from build123d import *

# Parameters (mm, degrees)
F8_DEPTH  = 54.8865515739
F1_DEPTH  = 36.7471762002
F3_DEPTH  = 25.4
F10_DEPTH = 62.1797274798
F4_DEPTH  = 13.1793599576
F5_F1_R   = 5.08
F5_F2_R   = 5.08


with BuildPart() as f8:
    # F6 (on Top) → F8 (new body)
    with BuildSketch(Plane.XY):
        Polygon((-47.3731532693, 49.1066724062), (-47.3731532693, -49.1066724062), (47.3731532693, -49.1066724062), (47.3731532693, 0), (0, 0), (0, 49.1066724062), align=None)
    extrude(amount=F8_DEPTH)

    # F0 (on face) → F1 (join)
    with BuildSketch(Plane.XY.offset(54.8865515739)):
        Polygon((0, 49.1066724062), (-23.6865766346, 49.1066724062), (-23.6865766346, -24.5533362031), (47.3731532693, -24.5533362031), (47.3731532693, 0), (0, 0), align=None)
    extrude(amount=-F1_DEPTH)

    # F2 (on face) → F3 (cut)
    with BuildSketch(Plane.XY.offset(54.8865515739)):
        Polygon((-23.6865766346, -24.5533362031), (47.3731532693, -24.5533362031), (47.3731532693, 0), (0, 0), (0, 49.1066724062), (-23.6865766346, 49.1066724062), align=None)
    extrude(amount=-F3_DEPTH, mode=Mode.SUBTRACT)

    # F9 (on face) → F10 (join)
    with BuildSketch(Plane.XY.offset(54.8865515739)):
        Polygon((0, -49.1066724062), (-0.0103376806, -24.5533362031), (-23.6865766346, -24.5533362031), (-23.6865766346, -19.0210193396), (-23.6865766346, 0), (-47.3731532693, 0), (-47.3731532693, -11.8761584163), (-47.3731532693, -49.1066724062), align=None)
    extrude(amount=F10_DEPTH)

    # F4 (cut): a face of the model
    f4_faces = [f8.faces().sort_by_distance(p)[0] for p in [
        (-27.6363494072, -28.6452612162, 117.0662790537),
    ]]
    extrude(f4_faces, amount=-F4_DEPTH, mode=Mode.SUBTRACT)

    # F5: fillet of radius 5.08 on 32 edges, made by hand

    # F5_f1
    f5_f1_edges = [f8.edges().sort_by_distance(p)[0] for p in [
        (-23.6865766346, -24.5533362031, 66.686735335),
        (-35.529864952, 0, 54.8865515739),
        (-0.0051688403, -36.8300043046, 54.8865515739),
        (11.8432883173, -24.5533362031, 29.4865515739),
        (-23.6865766346, 12.2766681015, 29.4865515739),
    ]]
    fillet(f5_f1_edges, radius=F5_F1_R)

    # F5_f2
    f5_f2_edges = [f8.edges().sort_by_distance(p)[0] for p in [
        (-0.0051688403, -36.8300043046, 103.8869190961),
        (-9.3084571576, -24.5533362031, 103.8869190961),
        (-23.6865766346, -9.7366681015, 103.8869190961),
        (-35.529864952, 0, 103.8869190961),
        (-47.3731532693, -24.5533362031, 103.8869190961),
        (-23.6865766346, -49.1066724062, 103.8869190961),
        (-0.0103376806, -24.5533362031, 81.926735335),
        (0, -49.1066724062, 81.926735335),
        (-23.6865766346, 0, 81.926735335),
        (-47.3731532693, 0, 81.926735335),
        (47.3731532693, -36.8300043046, 54.8865515739),
        (-35.529864952, 49.1066724062, 54.8865515739),
        (23.6865766346, 0, 0),
        (47.3731532693, -24.5533362031, 0),
        (47.3731532693, 0, 14.7432757869),
        (23.6865766346, 0, 29.4865515739),
        (47.3731532693, -9.7366681015, 29.4865515739),
        (0, 24.5533362031, 29.4865515739),
        (-9.3032883173, 49.1066724062, 29.4865515739),
        (0, 49.1066724062, 14.7432757869),
        (0, 24.5533362031, 0),
        (47.3731532693, -49.1066724062, 27.4432757869),
        (0, -49.1066724062, 0),
        (-47.3731532693, -49.1066724062, 51.9434595481),
        (-23.6865766346, 49.1066724062, 0),
        (-47.3731532693, 49.1066724062, 27.4432757869),
        (-47.3731532693, 0, 0),
        (-22.1986790831, 49.1066724062, 30.9744491254),
        (47.3731532693, -23.0654386515, 30.9744491254),
        (-47.3731532693, 1.4878975516, 56.3744491254),
        (-23.6865766346, 1.4878975516, 56.3744491254),
        (1.4878976834, -49.1066724062, 56.3744491254),
        (1.4775600029, -24.5533362031, 56.3744491254),
        (-22.1986790831, -23.0654386515, 103.8869190961),
    ]]
    fillet(f5_f2_edges, radius=F5_F2_R)


solid = f8.part
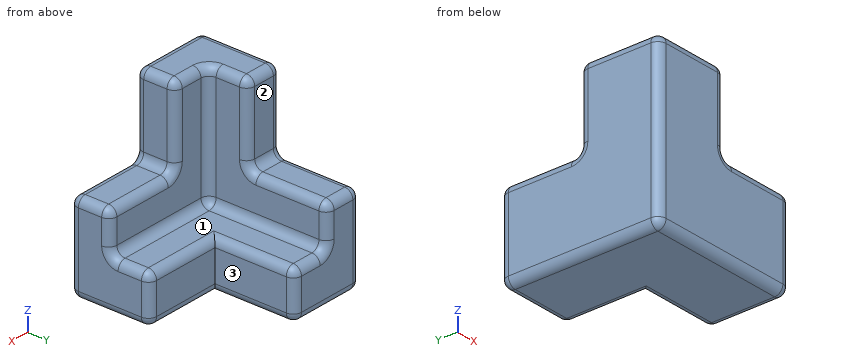
CAD build for the part. Positions are in the model's coordinates, mm. Face numbers are marked on the shaded views. A direction names the side the tool comes from. Coordinates: 2 decimals unless noted, no trailing zeros. Write each loop counter-clockwise with the first axis right and the second up, starting at its lowest first coordinate (ties: lowest second). Pieces come first, ordered by that corner, then holes. Notation, with made-up numbers: M 63.5,83.5 L 111.5,83.5 A24 cw 111.5,116.5 Z; hole C 87.25,74 d10. An arc over 180 degrees is marked long. Answer as a JSON object with one key per item and string values. Group by question number.
1) Pin check, flat tips, straight feed: pin 1 Ø16 at (y, z) = (-38, 74) entering from +X; pin 2 Ø18.5 at (x, z) = (21.5, 61.5) entering from +Y; pin 3 Ø10 at (x, y) = (-20.5, -27) entering from +Z; pin 4 Ø16 at (x, y) = (22.5, -33.5) entering from +Z. Stop position of each tip, or through.
2) Wall check: line 1 (Y direction, x = -42, z = 93); line 2 (Y direction, x = -16.5, z = 40); line 3 (Z direction, x = -42, y = 5.5). Give the ranges that are in metal, low to high. Write a range as from..to.
3) Saw through at B-B (y = 26.5). Write the cut outline in (x, z), plus the area to 3 significant figures.
4) Tool access for the marked faces 1, 2 and 3: list every direction of +Z, -Z, +X, -X, +Y, -Y with a clear straight run to the whole face (end or side of a thin tool).
5) Saw through at A-A (x = 14.5). Write the cut outline in (y, z), plus the area to 3 significant figures.
6) Saw through at C-C (z = 18.5). Write the cut outline in (x, y), plus the area to 3 significant figures.
Values follow:
{
 "1": {"pin 1": "stops at x = 0", "pin 2": "stops at y = -25.18", "pin 3": "stops at z = 103.89", "pin 4": "stops at z = 54.89"},
 "2": {"line 1": "y = -49.11..0", "line 2": "y = -49.11..-24.55", "line 3": "z = 0..54.89"},
 "3": {"outline": "M -47.37,5.08 A5.08 ccw -42.29,0 L -5.08,0 A5.08 ccw 0,5.08 L 0,24.41 A5.08 ccw -5.08,29.49 L -18.61,29.49 A5.08 cw -23.69,34.57 L -23.69,49.81 A5.08 ccw -28.77,54.89 L -42.29,54.89 A5.08 ccw -47.37,49.81 Z", "area": "1,980 mm2"},
 "4": {"face 1": "+Z, +X, +Y", "face 2": "+Z, +X, -X, +Y", "face 3": "+Z, -Z, +X, +Y"},
 "5": {"outline": "M -49.11,5.08 A5.08 ccw -44.03,0 L -5.08,0 A5.08 ccw 0,5.08 L 0,24.41 A5.08 ccw -5.08,29.49 L -19.47,29.49 A5.08 cw -24.55,34.57 L -24.55,49.81 A5.08 ccw -29.63,54.89 L -44.03,54.89 A5.08 ccw -49.11,49.81 Z", "area": "2,050 mm2"},
 "6": {"outline": "M -47.37,-44.03 A5.08 ccw -42.29,-49.11 L 42.29,-49.11 A5.08 ccw 47.37,-44.03 L 47.37,-5.08 A5.08 ccw 42.29,0 L 0,0 L 0,44.03 A5.08 ccw -5.08,49.11 L -42.29,49.11 A5.08 ccw -47.37,44.03 Z", "area": "6,950 mm2"}
}
